For this review, use the dimensioned drawing (mm, ordinates from the lowest corner) and the shaded views. Round coordinates to 2 decimals unless told otherwise and drop trailing zeros. Loops run counter-clockwise (first coordinate to the right, second up) from the corner with the lowest first, then second, coordinate; pieces in that order, holes last. Notation, with made-up numbers: M 65.5,20 L 122.5,20 A22 cw 122.5,52 Z; hole C -18,20.5 d6. An arc over 180 degrees is marked long. Answer as a JSON object with one key per item and string values. Group by question number.
Item 1: To check wall thickness, follow line 1 (X direction, y = 64.5, z = 2.5); line 2 (X direction, y = 7.5, z = 1.4) (1 decimal); line 3 (Y direction, x = 152.4, z = 1.7). State the ranges of each line that lie inside material, in increasing order.
Item 2: Consider section C-C (z = 2.4). State how many separate pieces and enclosed holes the cut face has, and give its area (3 significant figures).
Item 3: Consider section B-B (y = 69). Give the boundary of the cut face in (x, z) (1 decimal).
Item 4: Insertion check: P1, Ø1.6, axis at x = 4.5, z = 2, coming from the +Y side (1 decimal); P2, Ø1, axis at x = 301.5, z = 1, coming from the -Y side (1 decimal); P3, Ø1, axis at y = 86.5, z = 1.5, coming from the +X side (1 decimal). Each pin has a flat end and moves straight along its axis. Give the tip position at first contact, or say it passes through.
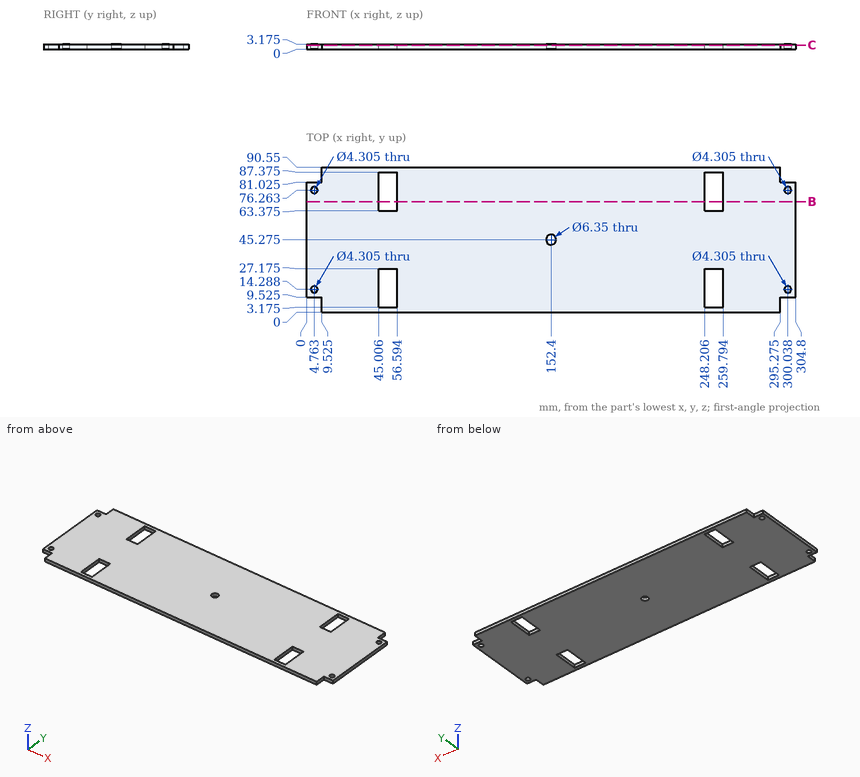
Geometry results:
{
 "1": {"line 1": "x = 0 to 45.01, 56.59 to 248.21, 259.79 to 304.8", "line 2": "x = 9.5 to 45, 56.6 to 248.2, 259.8 to 295.3", "line 3": "y = 0 to 42.1, 48.45 to 90.55"},
 "2": {"separate pieces": "1", "enclosed holes": "9", "area": "26,000 mm^2"},
 "3": {"outline": "M 0,0 L 45,0 L 45,3.2 L 0,3.2 Z; M 56.6,0 L 248.2,0 L 248.2,3.2 L 56.6,3.2 Z; M 259.8,0 L 304.8,0 L 304.8,3.2 L 259.8,3.2 Z"},
 "4": {"P1": "stops at y = 81", "P2": "stops at y = 9.5", "P3": "stops at x = 295.3"}
}
